Autodesk Inventor part; units mm, degrees
ref_plane "YZ Plane" through (0, 0, 0) normal (1, 0, 0) x (0, 1, 0)
ref_plane "XZ Plane" through (0, 0, 0) normal (0, 1, 0) x (-1, 0, 0)
ref_plane "XY Plane" through (0, 0, 0) normal (0, 0, 1) x (1, 0, 0)
sketch "Sketch1" plane through (0, 0, 0) normal (1, 0, 0) x (0, 1, 0)
  line L0 (0, 0) -> (50.8, 0)
  line L1 (0, 133.35) -> (0, 184.15)
  line L2 (0, 184.15) -> (29.2989, 184.15)
  line L3 (73.025, 184.15) -> (73.025, 133.35)
  line L4 (3.175, 180.975) -> (3.175, 136.525)
  line L5 (69.85, 136.525) -> (69.85, 180.975)
  line L6 (29.2989, 148.3694) -> (29.2989, 120.4477)
  line L7 (41.9989, 148.9666) -> (41.9989, 122.6874)
  line L8 (0, 133.35) -> (29.2989, 133.35)
  line L9 (41.9989, 133.35) -> (73.025, 133.35)
  line L10 (3.175, 136.525) -> (29.2989, 136.525)
  line L11 (41.9989, 136.525) -> (69.85, 136.525)
  line L12 (35.6489, 182.5625) -> (41.9989, 182.5625)
  line L13 (41.9989, 182.5625) -> (41.9989, 180.975)
  line L14 (35.6489, 182.5625) -> (29.2989, 182.5625)
  line L15 (29.2989, 182.5625) -> (29.2989, 184.15)
  line L16 (69.85, 180.975) -> (41.9989, 180.975)
  line L17 (35.6489, 180.975) -> (3.175, 180.975)
  line L18 (35.6489, 170.617) -> (35.6489, 180.975)
  line L19 (35.6489, 184.15) -> (35.6489, 201.7381)
  line L20 (35.6489, 180.975) -> (41.9989, 180.975)
  point P0 (3.175, 180.975)
  point P1 (69.85, 136.525)
  dimension "d0" = 50.8
  dimension "d3" = 50.8
  dimension "d4" = 73.025
  dimension "d5" = 3.175
  dimension "d6" = 3.175
  dimension "d7" = 3.175
  dimension "d8" = 3.175
  dimension "d9" = 3.175
  dimension "d11" = 3.175
  dimension "d13" = 26.1239
  dimension "d14" = 12.7
  dimension "d16" = 133.35
  dimension "d17" = 3.175
  dimension "d18" = 3.175
  dimension "d19" = 6.35
  dimension "d21" = 6.35
  dimension "d22" = 6.35
revolve "Revolution1" add sketch "Sketch1" angle 180 about axis through (0, 0, 0) along (0, 1, 0)
properties part number "Outer_Shell_Bottom"
Verification items for the finished model (mm, model axes). A direction names the side the tool comes from. Coordinates: 2 decimals unless noted, no trailing zeros. Order: outer loops, then holes, each group sorted by start corner. A loop starts at its lowest first (then second) coordinate and runs counter-clockwise, first axis right, second up. Notation, with made-up numbers: M 78,64 L 85,64 A13 ccw 85,73 Z; hole C 72.5,63.5 d8. An arc over 180 degrees is marked long. Write each question's results on one line, items separated by ' | '.
1) Section check A-A on y = 8. Record the cut outline in (x, z) (3 decimals).
Solved:
outline: M 0,-184.15 A184.15 ccw 0,184.15 L 0,180.975 A180.975 cw 0,-180.975 Z; M 0,-136.525 A136.525 ccw 0,136.525 L 0,133.35 A133.35 cw 0,-133.35 Z
2) Access from +Z, -Z, +X, -X, +Y, -Y to the whole of each face (thin tool, end or side, straight path). Record for faces 1 (the face through (138, 3.175, -14)), 2 (the face through (133.318, 14.855, 2.932)), 3 (the face through (134, 29.299, -1)), 4 (the face through (182.52, 35.56, -4.01)).
Solved:
face 1: +Y | face 2: -X, +Y, -Y | face 3: -X, +Y | face 4: +X, +Y
3) Section check C-C on x = 154.5. Record the cut outline in (y, z) (3 decimals), plus the area to 3 significant figures.
Solved:
outline: M 0,-100.205 L 29.299,-100.205 L 29.299,-97.256 L 41.999,-97.256 L 41.999,-94.243 L 3.175,-94.243 L 3.175,94.243 L 41.999,94.243 L 41.999,97.256 L 29.299,97.256 L 29.299,100.205 L 0,100.205 Z | area: 1,020 mm²
4) Scan lines: line 1 along Z through (x, y) = (103, 5.5); line 2 along Z through (x, y) = (63, 27.5); line 3 along Z through (x, y) = (83.5, 34). Record each from-to range of solid material in increasing order. Write a range as [from, to].
Solved:
line 1: z = [-152.65, -148.81], [-89.61, -84.69], [84.69, 89.61], [148.81, 152.65] | line 2: z = [-173.04, -169.66], [-121.12, -117.53], [117.53, 121.12], [169.66, 173.04] | line 3: z = [-162.35, -160.56], [160.56, 162.35]
5) Gauge pin test, flat ends, axial feed: pin 1 Ø1.5 at (x, z) = (122.5, 113.5) entering from +Y (3 decimals); pin 2 Ø1.5 at (y, z) = (20, 33) entering from +X; pin 3 Ø2 at (y, z) = (24.5, -75) entering from +X. Record the tip position at first contact, or that the pin passes through.
Solved:
pin 1: stops at y = 3.175 | pin 2: stops at x = 181.3 | pin 3: stops at x = 168.63
6) Release check for a two-part mould opening along Z. For faces 5 (the face through (136.492, 16.42, 3.002)), 6 (the face through (184.105, 14.855, 4.049)), 7 (the face through (0, 2, 163)), 8 (the face through (180.93, 22.86, 3.98)) record: pulls with the +Z half, pulls with the -Z half, needs draft (parallel to the pull), parting line crosses it, or undercut.
Solved:
face 5: undercut | face 6: parting line crosses it | face 7: needs draft | face 8: undercut
